Source: three-view drawing plus pictorial views. Frame: mm from the lowest corner of the part. A direction names the side the tool comes from. Give positions to 0.01 mm unless a question says otherwise; leave off trailing zeros. Loops run counter-clockwise (first coordinate to the right, second up) from the corner with the lowest first, then second, coordinate; pieces in that order, holes last. Notation, with made-up numbers: (-7, 42.25) -> (43, 42.25) arc R25 ccw to (43, 56.25) -> close; hole circle Ø3 at (-3, 72). An arc over 180 degrees is marked (long way). Answer as a JSON object with one key per item and string values. Group by question number.
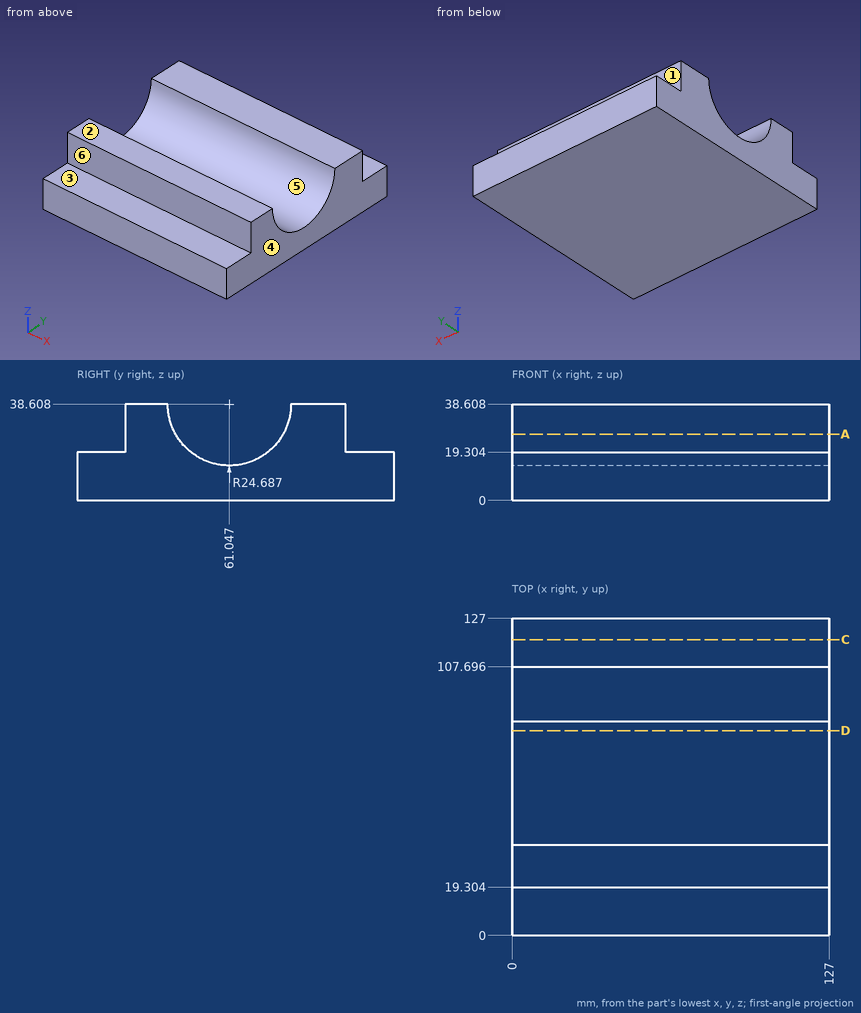
(1) Access query for the marked faces 1, 2 and 3. Directions: +Z, -Z, +X, -X, +Y, -Y. A direction counts if a zero-diameter tool reaches every point of the face in a straight line with its end or side. Return the directions, or none.
(2) Section query C-C on y = 118.5. Return the cut outline in (x, z).
(3) Mould query, pull axis Y, two halves, no side actions, for the marked faces 4, 5 and 6. Classes: pulls with the +Y half, pulls with the -Y half, needs draft (parallel to the pull), parting line crosses it, or undercut.
(4) First-contact query: pin 1 (1 mm diameter, centred on x = 98.5, z = 31.5, fed in from -Y); pin 2 (1.5 mm diameter, centred on x = 114, y = 109, fed in from +Z); pin 3 (15.5 mm diameter, centred on x = 51, z = 33.5, fed in from +Y). Flat tips, straight axial feed; report the tip coordinate or a pass-through.
(5) Material intervals for line 1 (Z direction, x = 79, y = 17); line 2 (Y direction, x = 32, z = 23.5) (1 decimal); line 3 (Y direction, x = 29.5, z = 20.5) (1 decimal), sorted ascending. Write a range as from..to.
(6) Section query D-D on y = 82. Return the cut outline in (x, z) (1 decimal), plus the area to 3 significant figures.
(7) Section query A-A on z = 26.5. Return the cut outline in (x, y).
Result:
{
 "1": {"face 1": "+Z, +X, -X, +Y", "face 2": "+Z, +X, -X, +Y, -Y", "face 3": "+Z, +X, -X, -Y"},
 "2": {"outline": "(0, 0) -> (127, 0) -> (127, 19.3) -> (0, 19.3) -> close"},
 "3": {"face 4": "needs draft", "face 5": "undercut", "face 6": "pulls with the -Y half"},
 "4": {"pin 1": "y = 19.3", "pin 2": "z = 19.3", "pin 3": "y = 107.7"},
 "5": {"line 1": "0..19.3", "line 2": "19.3..41.5, 80.6..107.7", "line 3": "19.3..44.3, 77.8..107.7"},
 "6": {"outline": "(0, 0) -> (127, 0) -> (127, 25.6) -> (0, 25.6) -> close", "area": "3,250 mm²"},
 "7": {"outline": "(0, 19.3) -> (127, 19.3) -> (127, 39.53) -> (0, 39.53) -> close; (0, 82.56) -> (127, 82.56) -> (127, 107.7) -> (0, 107.7) -> close"}
}
